Could you check a few things on this model? Use its own coordinates, in mm. Coordinates: 2 decimals unless noted, no trailing zeros. Write each loop counter-clockwise with the first axis right and the second up, starting at its lowest first coordinate (ties: lowest second). Pieces come first, ordered by that corner, then holes.
Item 1: If I drill on probe 1 along Z at (x, y) = (2, -1.25); probe 2 along Z at (x, y) = (1.25, 1.5); probe 3 along X at (y, z) = (-2.25, -5.5), over which ranges is the centre line in solid material (lowest first)?
Item 2: I want a section at A-A on y = -1.75. Please give me the cut outline in (x, z).
Item 3: I want a section at B-B on x = -3.5. Please give me the cut outline in (y, z), then the cut area to 3 significant figures.
from build123d import *
from build123d.topology import SkipClean

# Parameters (mm, degrees)
SALIENTE_EXTRUIR1_DEPTH = 1
SALIENTE_EXTRUIR2_DEPTH = 7
CROQUIS4_W              = 21.763285414
CROQUIS4_H              = 20.505608116
CORTAR_EXTRUIR1_DEPTH   = 14


with BuildPart() as part:
    # Croquis1 → Saliente-Extruir1 (new body)
    with BuildSketch(Plane.XY):
        with BuildLine():
            Line((-4, 4), (4, 4))
            ThreePointArc((4, 4), (4.707106781, 3.707106781), (5, 3))
            Line((5, 3), (5, -3))
            ThreePointArc((5, -3), (4.707106781, -3.707106781), (4, -4))
            Line((4, -4), (-4, -4))
            ThreePointArc((-4, -4), (-4.707106781, -3.707106781), (-5, -3))
            Line((-5, -3), (-5, 3))
            ThreePointArc((-5, 3), (-4.707106781, 3.707106781), (-4, 4))
        make_face()
    extrude(amount=-SALIENTE_EXTRUIR1_DEPTH)

    # Croquis2 → Saliente-Extruir2 (add, symmetric)
    with BuildSketch(Plane(origin=(0, 0, 0), x_dir=(1, 0, 0), z_dir=(0, 1, 0))):
        with BuildLine():
            Line((0, 1), (-6, 1))
            ThreePointArc((-6, 1), (-4.242640667, 5.242640684), (0, 7))
            ThreePointArc((0, 7), (4.242640687, 5.242640687), (6, 1))
            Line((6, 1), (0, 1))
        make_face()
    extrude(amount=SALIENTE_EXTRUIR2_DEPTH, both=True)

    # Croquis4 → Cortar-Extruir1 (cut)
    with SkipClean():  # the faces are left unmerged after this step: merging them gives an invalid solid
        with BuildSketch(Plane.XY):
            with Locations((0.374231366, -0.207273628)):
                Rectangle(CROQUIS4_W, CROQUIS4_H)
            with BuildLine():
                Line((5, -3), (5, 3))
                ThreePointArc((5, 3), (4.707106781, 3.707106781), (4, 4))
                Line((4, 4), (-4, 4))
                ThreePointArc((-4, 4), (-4.707106781, 3.707106781), (-5, 3))
                Line((-5, 3), (-5, -3))
                ThreePointArc((-5, -3), (-4.707106781, -3.707106781), (-4, -4))
                Line((-4, -4), (4, -4))
                ThreePointArc((4, -4), (4.707106781, -3.707106781), (5, -3))
            make_face(mode=Mode.SUBTRACT)
        extrude(amount=-CORTAR_EXTRUIR1_DEPTH, mode=Mode.SUBTRACT)
    add(part.part.scale(1), mode=Mode.REPLACE)  # the faces are merged on a copy


solid = part.part
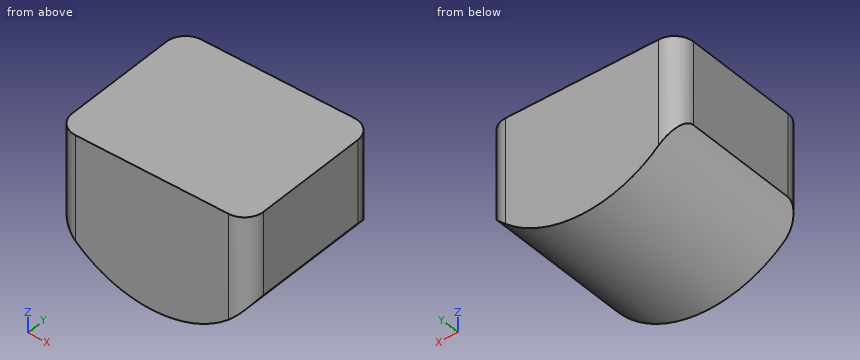
Response values:
1. probe 1: z = -6.66 to 0
1. probe 2: z = -6.87 to 0
1. probe 3: x = -3.97 to 3.97
2. outline: (-5, -4.32) arc R6 ccw to (5, -4.32) - (5, 0) - (-5, 0) - close
3. outline: (-4, -5.87) - (4, -5.87) - (4, 0) - (-4, 0) - close
3. area: 47.0 mm2
